Could you check a few things on this drawing? It's one solid part, dimensions in mm from its lowest x, y, z. A direction names the side the tool comes from. Round coordinates to 2 decimals unless told otherwise and drop trailing zeros. Write each loop counter-clockwise with the first axis right and the second up, starting at its lowest first coordinate (ties: lowest second). Pieces come first, ordered by that corner, then holes. Notation, with made-up numbers: (9.25, -26.75) -> (42.25, -26.75) arc R20 cw to (42.25, -7.75) -> close; hole circle Ø10 at (60.5, -7.75). An arc over 180 degrees is marked (long way). Answer in a Markdown table with one row per item.
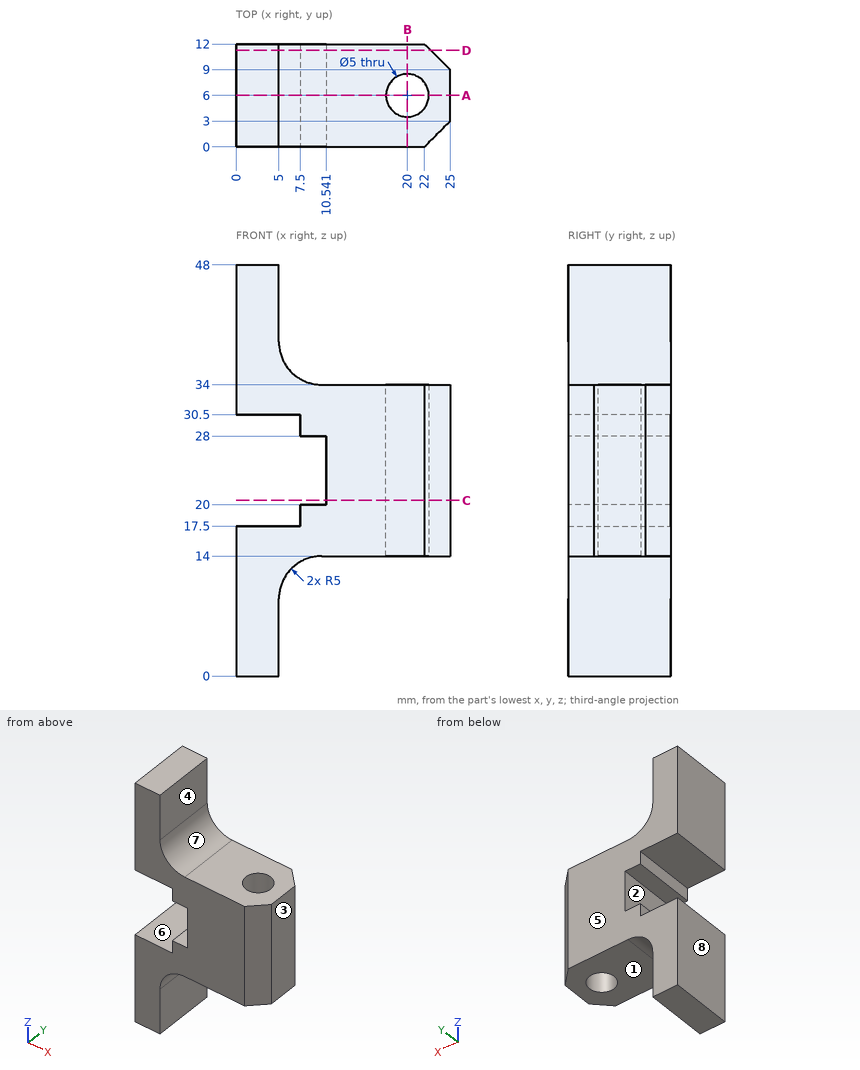
1) Thinking about a two-plate mould opening in Z: for the marked faces 6, 7 and 8, which applies, +Z half, -Z half, draft (parallel to the pull), parting line (faces both ways), or undercut?
Findings:
| item | result |
|---|---|
| face 6 | undercut |
| face 7 | +Z half |
| face 8 | draft |
2) Imagine slicing it at B-B, the plane x = 20. Please give me the cut outline in (y, z), plus the area to 3 significant figures.
Findings:
| item | result |
|---|---|
| outline | (0, 14) -> (3.5, 14) -> (3.5, 34) -> (0, 34) -> close; (8.5, 14) -> (12, 14) -> (12, 34) -> (8.5, 34) -> close |
| area | 140 mm^2 |
3) Please list where these lines run through material, in increasing order: line 1 (Y direction, x = 20, z = 27.5); line 2 (Z direction, x = 4, y = 7.5); line 3 (X direction, y = 1.5, z = 40.5).
Findings:
| item | result |
|---|---|
| line 1 | y = 0 to 3.5, 8.5 to 12 |
| line 2 | z = 0 to 17.5, 30.5 to 48 |
| line 3 | x = 0 to 5 |
4) Imagine slicing it at A-A, the plane y = 6. Please give me the cut outline in (x, z).
Findings:
| item | result |
|---|---|
| outline | (0, 0) -> (5, 0) -> (5, 9) arc R5 cw to (10, 14) -> (17.5, 14) -> (17.5, 34) -> (10, 34) arc R5 cw to (5, 39) -> (5, 48) -> (0, 48) -> (0, 30.5) -> (7.5, 30.5) -> (7.5, 28) -> (10.54, 28) -> (10.54, 20) -> (7.5, 20) -> (7.5, 17.5) -> (0, 17.5) -> close; (22.5, 14) -> (25, 14) -> (25, 34) -> (22.5, 34) -> close |
5) Imagine slicing it at D-D, the plane y = 11.25. Please give me the cut outline in (x, z).
Findings:
| item | result |
|---|---|
| outline | (0, 0) -> (5, 0) -> (5, 9) arc R5 cw to (10, 14) -> (22.75, 14) -> (22.75, 34) -> (10, 34) arc R5 cw to (5, 39) -> (5, 48) -> (0, 48) -> (0, 30.5) -> (7.5, 30.5) -> (7.5, 28) -> (10.54, 28) -> (10.54, 20) -> (7.5, 20) -> (7.5, 17.5) -> (0, 17.5) -> close |
6) For the marked faces 1, 2, 3, 4 and 5, which set-ups out of +Z, -Z, +X, -X, +Y, -Y let a thin tool reach every point of the face, with its end or its side?
Findings:
| item | result |
|---|---|
| face 1 | -Z, +X, +Y, -Y |
| face 2 | -X, +Y, -Y |
| face 3 | +Z, -Z, +X, +Y, -Y |
| face 4 | +Z, +X, +Y, -Y |
| face 5 | +Z, -Z, +X, -X, +Y |
7) Imagine slicing it at C-C, the plane z = 20.5. Please give me the cut outline in (x, y).
Findings:
| item | result |
|---|---|
| outline | (10.54, 0) -> (22, 0) -> (25, 3) -> (25, 9) -> (22, 12) -> (10.54, 12) -> close; hole circle Ø5 at (20, 6) |
8) For pin 1 (2 mm diameter, centred on y = 2.5, z = 20, fed in from +X); pin 2 (6 mm diameter, centred on x = 9, y = 10.5, fed in from -Z); pin 3 (0.8 mm diameter, centred on y = 4, z = 19.5, fed in from -X); pin 4 (7 mm diameter, centred on y = 7, z = 45.5, fed in from +X), each with a flat end and sliding along its axis, tell me the tip position at first contact or that it passes through.
Findings:
| item | result |
|---|---|
| pin 1 | stops at x = 25 |
| pin 2 | stops at z = 12 |
| pin 3 | stops at x = 7.5 |
| pin 4 | stops at x = 5 |
